from build123d import *

# Parameters (mm, degrees)
SKETCH1_R           = 3.5
SKETCH1_R_2         = 2.4
BOSS_EXTRUDE1_DEPTH = 6
SKETCH1_2_R         = 2.4
BOSS_EXTRUDE2_DEPTH = 1
FILLET1_R           = 1.5
CHAMFER1_SIZE       = 0.5


with BuildPart() as part:
    # Sketch1 → Boss-Extrude1 (new body)
    with BuildSketch(Plane.XY):
        Circle(SKETCH1_R)
        Circle(SKETCH1_R_2, mode=Mode.SUBTRACT)
    extrude(amount=BOSS_EXTRUDE1_DEPTH)

    # Sketch1<2> → Boss-Extrude2 (add)
    with BuildSketch(Plane.XY):
        Circle(SKETCH1_2_R)
    extrude(amount=BOSS_EXTRUDE2_DEPTH)

    # Fillet1
    fillet1_edges = [part.edges().sort_by_distance(p)[0] for p in [
        (-3.5, 0, 0),
    ]]
    fillet(fillet1_edges, radius=FILLET1_R)

    # Chamfer1
    chamfer1_edges = [part.edges().sort_by_distance(p)[0] for p in [
        (-2.4, 0, 6),
    ]]
    chamfer(chamfer1_edges, length=CHAMFER1_SIZE)


solid = part.part
Can you work these out from the model? Positions are in its coordinate system, mm. A direction names the side the tool comes from. Give positions to 0.01 mm unless a question says otherwise; leave off trailing zeros. Order: outer loops, then holes, each group sorted by start corner. A loop starts at its lowest first (then second) coordinate and runs counter-clockwise, first axis right, second up. Notation, with made-up numbers: M 38,49.25 L 58,49.25 A21 cw 58,65.25 Z; hole C -22.75,22 d4. An arc over 180 degrees is marked long. Use a Markdown table: item, result. Add a question column.
Item 1: Suppose I cut it at B-B (z = 1.9). List the corners of the cut face in (x, y) for me.
Item 2: We'd pull the mould along X, two halves only. Please class faces 3 (the cylindrical face through (3.233, -1.341, 3.718)), 4 (the flat face through (0, 0, 0)), 5 (the cylindrical face through (1.29, 2.024, 3.218)): +X half, -X half, draft (parallel to the pull), parting line (faces both ways), or undercut.
Item 3: Suppose I cut it at A-A (x = 0). List the corners of the cut face in (y, z) for me, then the cut area to 3 significant figures.
Item 4: If I drill on L1, parallel to Y at x = 0, z = 4.25; L2, parallel to Z at x = 1.25, y = -1; L3, parallel to X at y = 1, z = 3.6, over which ranges is the centre line in solid material (lowest first)? Write a range as [from, to].
Item 5: Will this pin go through, and if not, where does the flat tip stop? pin 1 (2.5 mm diameter, centred on x = -0.5, y = -1, fed in from +Z).
Item 6: For faces 1 (the flat face through (-1, 3, 6)), 2 (the flat face through (0, 0, 1)), which set-ups out of +Z, -Z, +X, -X, +Y, -Y let a thin tool reach every point of the face, with its end or its side?
Answer sheet:
| question | item | result |
|---|---|---|
| 1 | outline | C 0,0 d7; hole C 0,0 d4.8 |
| 2 | face 3 | parting line |
| 2 | face 4 | draft |
| 2 | face 5 | undercut |
| 3 | outline | M -3.5,1.5 A1.5 ccw -2,0 L 2,0 A1.5 ccw 3.5,1.5 L 3.5,6 L 2.9,6 L 2.4,5.5 L 2.4,1 L -2.4,1 L -2.4,5.5 L -2.9,6 L -3.5,6 Z |
| 3 | area | 16.8 mm² |
| 4 | L1 | y = [-3.5, -2.4], [2.4, 3.5] |
| 4 | L2 | z = [0, 1] |
| 4 | L3 | x = [-3.35, -2.18], [2.18, 3.35] |
| 5 | pin 1 | stops at z = 1 |
| 6 | face 1 | +Z, +X, -X, +Y, -Y |
| 6 | face 2 | +Z |
